Verification items for this drawing (mm, ordinates from the low corner). A direction names the side the tool comes from. Round coordinates to 2 decimals unless told otherwise and drop trailing zeros. Write each loop counter-clockwise with the first axis right and the second up, starting at its lowest first coordinate (ties: lowest second). Pieces come first, ordered by that corner, then holes. Notation, with made-up numbers: (57.5, 88) -> (93.5, 88) arc R22 ccw to (93.5, 110) -> close; hole circle Ø4 at (58.25, 87.5). An arc over 180 degrees is marked (long way). One line per item, written item: value.
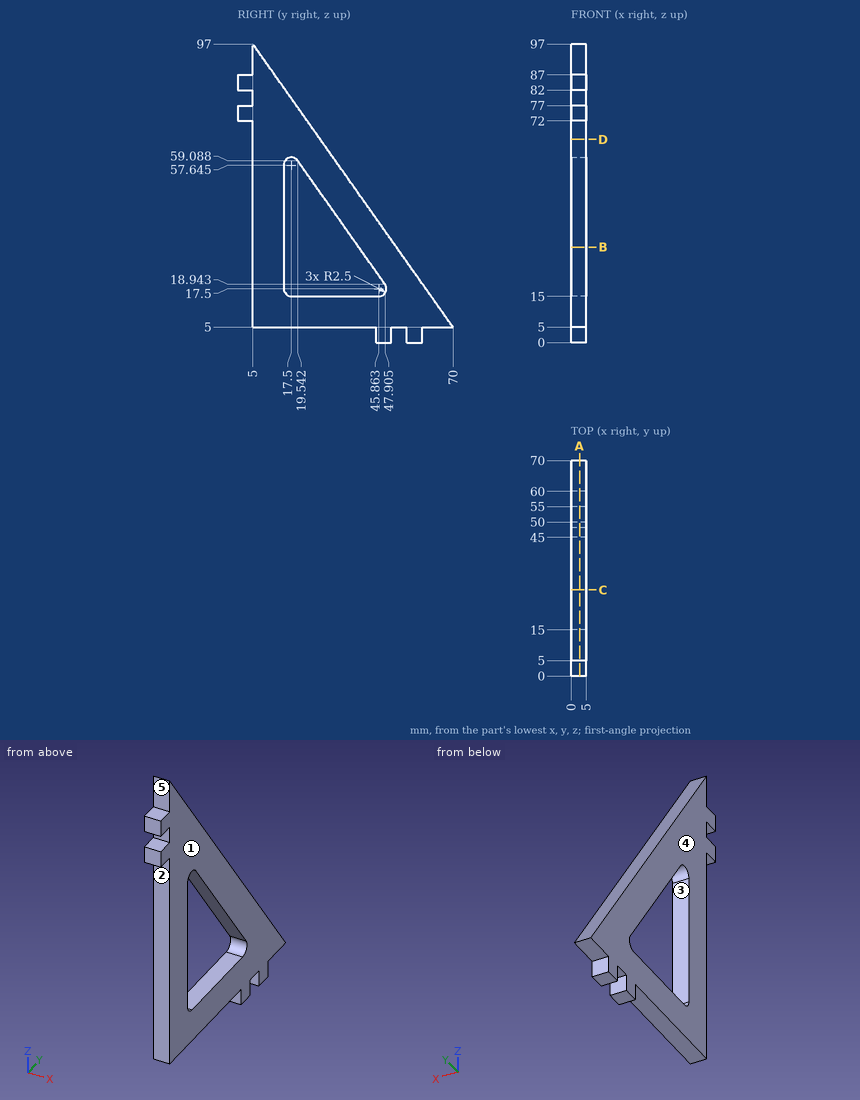
Item 1: Sectioned sample at A-A (x = 2.8). Enter the section's corners in (y, z) (1 decimal).
Result set:
outline: (0, 72) -> (5, 72) -> (5, 5) -> (45, 5) -> (45, 0) -> (50, 0) -> (50, 5) -> (55, 5) -> (55, 0) -> (60, 0) -> (60, 5) -> (70, 5) -> (5, 97) -> (5, 87) -> (0, 87) -> (0, 82) -> (5, 82) -> (5, 77) -> (0, 77) -> close; hole (15, 17.5) arc R2.5 ccw to (17.5, 15) -> (45.9, 15) arc R2.5 ccw to (47.9, 18.9) -> (19.5, 59.1) arc R2.5 ccw to (15, 57.6) -> close
Item 2: Material ranges on line 1 along Y through (x, z) = (0.5, 18) (1 decimal); line 2 along Z through (x, y) = (0.85, 41) (1 decimal); line 3 along Y through (x, z) = (3.8, 56) (1 decimal), recorded low to high.
Result set:
line 1: 5 to 15, 48.3 to 60.8
line 2: 5 to 15, 28.7 to 46
line 3: 5 to 15, 21.7 to 34
Item 3: Sectioned sample at D-D (z = 66). Enter the section's corners in (x, y).
Result set:
outline: (0, 5) -> (5, 5) -> (5, 26.9) -> (0, 26.9) -> close
Item 4: Sectioned sample at B-B (z = 31). Enter the section's corners in (x, y), then the cut area to 3 significant figures.
Result set:
outline: (0, 5) -> (5, 5) -> (5, 15) -> (0, 15) -> close; (0, 39.39) -> (5, 39.39) -> (5, 51.63) -> (0, 51.63) -> close
area: 111 mm^2
Item 5: Release check for a two-part mould opening along Y. For the marked faces 3, 4 and 5 record: pulls with the +Y half, pulls with the -Y half, needs draft (parallel to the pull), parting line crosses it, or undercut.
Result set:
face 3: undercut
face 4: needs draft
face 5: pulls with the -Y half
Item 6: Tool access check on the marked faces 1 and 2. Record the directions out of +Z, -Z, +X, -X, +Y, -Y that give a thin tool (end or side, any length) a straight path to the whole face; none if there is none.
Result set:
face 1: +Z, -Z, +X, +Y, -Y
face 2: -Z, +X, -X, -Y
Item 7: Sectioned sample at C-C (y = 28). Enter the section's corners in (x, z).
Result set:
outline: (0, 5) -> (5, 5) -> (5, 15) -> (0, 15) -> close; (0, 47.12) -> (5, 47.12) -> (5, 64.45) -> (0, 64.45) -> close
Item 8: Depth check by flat-ended pin: pin 1 (2.5 mm diameter, centred on x = 3.5, y = 2.5, fed in from +Z); pin 2 (1.5 mm diameter, centred on x = 2, y = 35.5, fed in from +Z); pin 3 (1.5 mm diameter, centred on x = 3.5, y = 53.5, fed in from -Z). Enter the tip coordinate at first touch or a pass-through.
Result set:
pin 1: z = 87
pin 2: z = 54.89
pin 3: z = 5
